Build history of the part. All positions in model axes, mm. Face numbers are marked on the shaded views. Give positions to 0.01 mm unless a question says otherwise; leave off trailing zeros. Order: outer loops, then holes, each group sorted by start corner. A loop starts at its lowest first (then second) coordinate and runs counter-clockwise, first axis right, second up. Notation, with made-up numbers: (6, -28) - (61, -28) arc R3 cw to (61, -23) - close; hole circle Ø11 at (78.5, -1). An arc over 180 degrees is marked (long way). Use a Markdown table: item, result. Add a question column.
(1) Mould opens along X. For the marked faces 1, 2 and 3 say: +X half, -X half, draft (parallel to the pull), parting line (faces both ways), or undercut.
(2) Flat gauge pins, fed straight in: pin 1 (4 mm diameter, centred on y = 12.5, z = 3, fed in from -X); pin 2 (4.5 mm diameter, centred on y = -14, z = 9, fed in from +X); pin 3 (2 mm diameter, centred on x = -13.5, y = 3.5, fed in from +Z); pin 4 (8 mm diameter, centred on y = 0.5, z = 9.5, fed in from -X). Where does each tip first touch, or does it go through?
(3) Wall check: line 1 (X direction, y = 0, z = 1.15); line 2 (X direction, y = 6.5, z = 6.75); line 3 (Z direction, x = -14, y = -5.5). Give the ranges that are in metal, low to high.
(4) Slice it at D-D (y = -15). Write the cut outline in (x, z), then the cut area to 3 significant figures.
(5) Slice it at A-A (y = -4). Write the cut outline in (x, z), then the cut area to 3 significant figures.
(6) Slice it at C-C (z = 1.5). Write the cut outline in (x, y).
(7) Slice it at B-B (x = -1). Write the cut outline in (y, z), then the cut area to 3 significant figures.
from build123d import *

# Parameters (mm, degrees)
F1_DEPTH = 3
F2_DEPTH = 15


with BuildPart() as f1:
    # F0 (on Top) → F1 (new body)
    with BuildSketch(Plane.XY):
        with BuildLine():
            ThreePointArc((0, -12.5), (-8.8388347648, 8.8388347648), (12.5, 0))
            ThreePointArc((12.5, 0), (11.5484941564, -4.7835429046), (8.8388347648, -8.8388347648))
            Line((8.8388347648, -8.8388347648), (10.9601551084, -10.9601551084))
            ThreePointArc((10.9601551084, -10.9601551084), (14.3201327539, -5.9315932017), (15.5, 0))
            ThreePointArc((15.5, 0), (-10.9601551084, 10.9601551084), (0, -15.5))
            Line((0, -15.5), (0, -12.5))
        make_face()
    extrude(amount=F1_DEPTH)

    # F0 (on Top) → F2 (join)
    with BuildSketch(Plane.XY):
        with BuildLine():
            Line((0, -18), (0, -15.5))
            ThreePointArc((0, -15.5), (-10.9601551084, 10.9601551084), (15.5, 0))
            ThreePointArc((15.5, 0), (14.3201327539, -5.9315932017), (10.9601551084, -10.9601551084))
            Line((10.9601551084, -10.9601551084), (12.7279220614, -12.7279220614))
            ThreePointArc((12.7279220614, -12.7279220614), (16.6298315852, -6.8883017826), (18, 0))
            ThreePointArc((18, 0), (-12.7279220614, 12.7279220614), (0, -18))
        make_face()
    extrude(amount=F2_DEPTH)


solid = f1.part
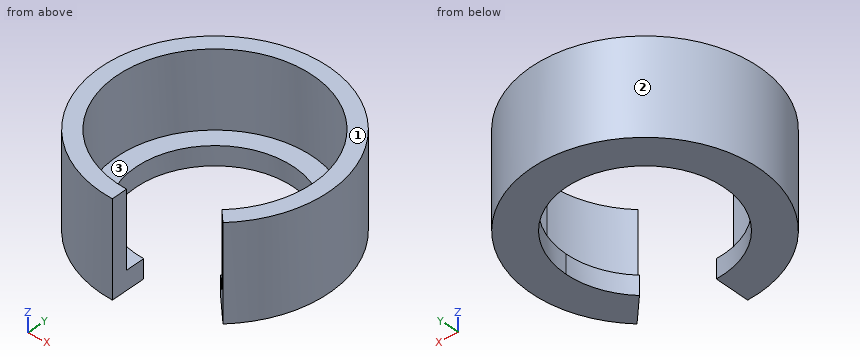
Solution:
| question | item | result |
|---|---|---|
| 1 | face 1 | draft |
| 1 | face 2 | parting line |
| 1 | face 3 | undercut |
| 2 | pin 1 | x = -14.62 |
| 2 | pin 2 | x = 13.64 |
| 2 | pin 3 | z = 3 |
| 2 | pin 4 | x = -18 |
| 3 | line 1 | -18 to -12.5, 12.5 to 18 |
| 3 | line 2 | -16.79 to -14.07, 14.07 to 16.79 |
| 3 | line 3 | 0 to 3 |
| 4 | outline | (-9.95, 0) - (0, 0) - (0, 3) - (-3.91, 3) - (-3.91, 15) - (-9.95, 15) - close |
| 4 | area | 102 mm2 |
| 5 | outline | (-17.55, 0) - (-11.84, 0) - (-11.84, 3) - (-14.97, 3) - (-14.97, 15) - (-17.55, 15) - close; (11.84, 0) - (17.55, 0) - (17.55, 15) - (14.97, 15) - (14.97, 3) - (11.84, 3) - close |
| 5 | area | 96.0 mm2 |
| 6 | outline | (0, -18) - (0, -12.5) arc R12.5 cw (long way) to (8.84, -8.84) - (12.73, -12.73) arc R18 ccw (long way) to start |
| 7 | outline | (-17.97, 0) - (-12.46, 0) - (-12.46, 3) - (-15.47, 3) - (-15.47, 15) - (-17.97, 15) - close; (12.46, 0) - (17.97, 0) - (17.97, 15) - (15.47, 15) - (15.47, 3) - (12.46, 3) - close |
| 7 | area | 93.2 mm2 |
